The model under review builds one solid part; all positions refer to its coordinate system, in mm. Round coordinates to 2 decimals unless told otherwise and drop trailing zeros. Write each loop counter-clockwise with the first axis right and the second up, starting at its lowest first coordinate (ties: lowest second). Pieces come first, ordered by that corner, then holes. Notation, with made-up numbers: (63.25, 83.25) - (121.25, 83.25) arc R23 ccw to (121.25, 104.25) - close; hole circle Ø5 at (-21.75, 13). An arc over 180 degrees is marked (long way). Use one line per item in the form item = value.
from build123d import *

# Parameters (mm, degrees)
BOSS_EXTRUDE1_DEPTH = 6.35
FILLET1_R           = 12.7
SKETCH2_R           = 2.286
CUT_EXTRUDE1_DEPTH  = 127.107467202
SKETCH3_R           = 3.81
CUT_EXTRUDE2_DEPTH  = 127.107467202
FILLET2_R           = 17.78


with BuildPart() as part:
    # Sketch1 → Boss-Extrude1 (new body)
    with BuildSketch(Plane(origin=(0, 0, 0), x_dir=(1, 0, 0), z_dir=(0, 1, 0))):
        with BuildLine():
            Line((0, 0), (92.075, 0))
            Line((92.075, 0), (92.075, 85.93582))
            ThreePointArc((92.075, 85.93582), (53.210726842, 46.653837999), (0, 31.75))
            Line((0, 31.75), (0, 0))
        make_face()
    extrude(amount=BOSS_EXTRUDE1_DEPTH)

    # Fillet1
    fillet1_edges = [part.edges().sort_by_distance(p)[0] for p in [
        (0, 3.175, -31.75),
    ]]
    fillet(fillet1_edges, radius=FILLET1_R)

    # Sketch2 → Cut-Extrude1 (cut, through all)
    with BuildSketch(Plane(origin=(0, 6.35, 0), x_dir=(1, 0, 0), z_dir=(0, 1, 0))):
        with Locations(Location((84.1375, 7.62, 0), (0, 0, 270))):
            Circle(SKETCH2_R)
        with Locations(Location((84.1375, 33.02, 0), (0, 0, 270))):
            Circle(SKETCH2_R)
    extrude(amount=-CUT_EXTRUDE1_DEPTH, mode=Mode.SUBTRACT)

    # Sketch3 → Cut-Extrude2 (cut, through all)
    with BuildSketch(Plane(origin=(0, 6.35, 0), x_dir=(1, 0, 0), z_dir=(0, 1, 0))):
        with Locations(Location((28.956, 18.288, 0), (0, 0, 270))):
            Circle(SKETCH3_R)
    extrude(amount=-CUT_EXTRUDE2_DEPTH, mode=Mode.SUBTRACT)

    # Fillet2
    fillet2_edges = [part.edges().sort_by_distance(p)[0] for p in [
        (92.075, 3.175, -85.93582),
    ]]
    fillet(fillet2_edges, radius=FILLET2_R)


solid = part.part
(1) Add section D-D on x = 80.5. Write out the cut boundary in (y, z).
Geometry results:
outline = (0, -56.07) - (6.35, -56.07) - (6.35, 0) - (0, 0) - close
(2) The part is to be moulded in two halves that separate along X. For faces 1 (the cylindrical face through (39.16, 3.131, -39.705)), 2 (the flat face through (56, 6.35, -23)), 3 (the cylindrical face through (25.576, 3.219, -16.53)), say which applies: +X half, -X half, draft (parallel to the pull), parting line (faces both ways), or undercut.
Geometry results:
face_1 = -X half
face_2 = draft
face_3 = undercut
(3) Add section C-C on y = 2.75. Count the separate pieces of the cut face and the enclosed holes in it, then the cut area to 3 significant figures.
Geometry results:
separate_pieces = 1
enclosed_holes = 3
area = 3,910 mm2
(4) To check wall thickness, follow L1, parallel to X at y = 2.75, z = -7.62 (1 decimal); L2, parallel to Z at x = 29.5, y = 4; L3, parallel to X at y = 1.5, z = -9 (3 decimals). State the ranges of each line that lie inside material, in increasing order.
Geometry results:
L1 = 0 to 81.9, 86.4 to 92.1
L2 = -36.3 to -22.06, -14.52 to 0
L3 = 0 to 82.315, 85.96 to 92.075
(5) Add section B-B on x = 30. Write out the cut boundary in (y, z).
Geometry results:
outline = (0, -36.45) - (6.35, -36.45) - (6.35, -21.95) - (0, -21.95) - close; (0, -14.62) - (6.35, -14.62) - (6.35, 0) - (0, 0) - close
(6) Insertion check: P1, Ø10, axis at x = 28.956, z = -18.288, coming from the -Y side; P2, Ø2, axis at x = 64, y = 3, coming from the -Z side; P3, Ø1, axis at y = 5.5, z = -46, coming from the -X side. Each pin has a flat end and moves straight along its axis. Give the tip position at first contact, or say it passes through.
Geometry results:
P1 = 0
P2 = -54.56
P3 = 51.2
